Here's the drawing with two shaded views (mm, measured from the low corner). I have some questions. A direction names the side the tool comes from. Give positions to 0.01 mm unless a question says otherwise; leave off trailing zeros. Order: outer loops, then holes, each group sorted by start corner. A loop starts at its lowest first (then second) coordinate and runs counter-clockwise, first axis right, second up. Notation, with made-up numbers: M -0.75,49 L 45.25,49 A23 ccw 45.25,62 Z; hole C -28.75,89.5 d8. An arc over 180 degrees is marked long. Write each question's results on one line, items separated by ' | '.
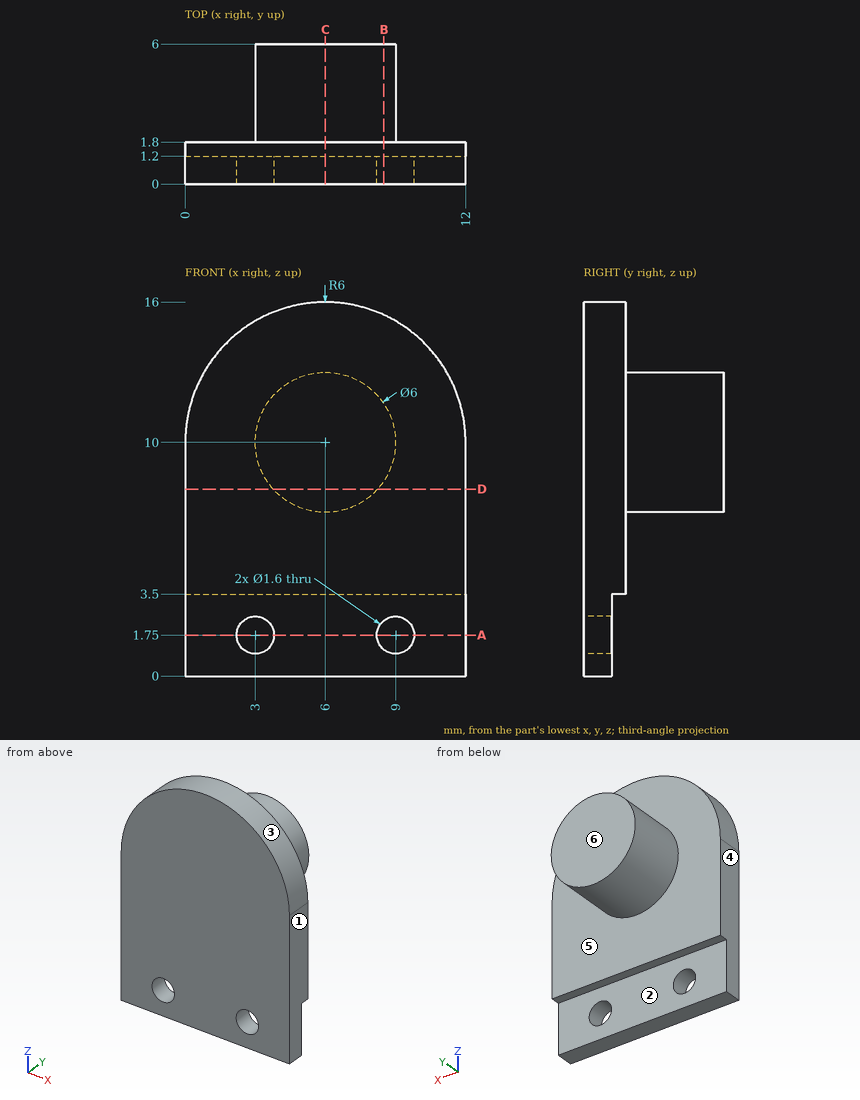
(1) Imagine slicing it at D-D, the plane z = 8. Write out the boundary of the cut face in (x, y).
Data:
outline: M 0,0 L 12,0 L 12,1.8 L 8.24,1.8 L 8.24,6 L 3.76,6 L 3.76,1.8 L 0,1.8 Z
(2) Imagine slicing it at B-B, the plane x = 8.5. Write out the boundary of the cut face in (y, z), plus the area to 3 significant figures.
Data:
outline: M 0,0 L 1.2,0 L 1.2,1.13 L 0,1.13 Z; M 0,2.37 L 1.2,2.37 L 1.2,3.5 L 1.8,3.5 L 1.8,8.34 L 6,8.34 L 6,11.66 L 1.8,11.66 L 1.8,15.45 L 0,15.45 Z | area: 38.1 mm2
(3) For the marked faces 5 and 6, which set-ups out of +Z, -Z, +X, -X, +Y, -Y let a thin tool reach every point of the face, with its end or its side?
Data:
face 5: +Y | face 6: +Z, -Z, +X, -X, +Y
(4) I need wall thicknesses on L1, parallel to X at y = 0.95, z = 1.75; L2, parallel to Y at x = 9.75, z = 2.5; L3, parallel to Y at x = 9.25, z = 11. Which ranges of each line are inside material? Lowest first, please. Write a range as from..to.
Data:
L1: x = 0..2.2, 3.8..8.2, 9.8..12 | L2: y = 0..1.2 | L3: y = 0..1.8
(5) Imagine slicing it at C-C, the plane x = 6. Write out the boundary of the cut face in (y, z).
Data:
outline: M 0,0 L 1.2,0 L 1.2,3.5 L 1.8,3.5 L 1.8,7 L 6,7 L 6,13 L 1.8,13 L 1.8,16 L 0,16 Z
(6) Will these pins go through, and if not, where does the flat tip stop? P1, Ø3, axis at x = 5, z = 1, coming from the +Y side; P2, Ø1, axis at y = 3, z = 9.5, coming from the -X side; P3, Ø0.5, axis at x = 6.5, y = 1.5, coming from the -Z side.
Data:
P1: stops at y = 1.2 | P2: stops at x = 3 | P3: stops at z = 3.5
(7) We'd pull the mould along X, two halves only. Please class the marked faces 1, 2, 3 and 4: +X half, -X half, draft (parallel to the pull), parting line (faces both ways), or undercut.
Data:
face 1: +X half | face 2: draft | face 3: parting line | face 4: -X half
(8) Imagine slicing it at A-A, the plane z = 1.75. Write out the boundary of the cut face in (x, y), plus the area to 3 significant figures.
Data:
outline: M 0,0 L 2.2,0 L 2.2,1.2 L 0,1.2 Z; M 3.8,0 L 8.2,0 L 8.2,1.2 L 3.8,1.2 Z; M 9.8,0 L 12,0 L 12,1.2 L 9.8,1.2 Z | area: 10.6 mm2
